For this review, take the finished solid that the model builds, in its own axes (mm). Face numbers are marked on the shaded views. A direction names the side the tool comes from. Round coordinates to 2 decimals unless told otherwise and drop trailing zeros. Write each loop counter-clockwise with the first axis right and the second up, starting at its lowest first coordinate (ties: lowest second). Pieces come first, ordered by that corner, then holes. Notation, with made-up numbers: (60, 31.25) - (100, 31.25) arc R9 ccw to (100, 38.25) - close; hole circle Ø10 at (-9, 67). An arc over 180 degrees is marked (long way). One line per item, written item: value. Start each with the question number.
Q1. Add section D-D on z = -13.5. Write out the cut boundary in (x, y), and give its area (3 significant figures).
Q2. Add section C-C on x = -16. Write out the cut boundary in (y, z), and give its area (3 significant figures).
Q3. Add section A-A on z = 0. Write out the cut boundary in (x, y), and give its area (3 significant figures).
Q4. Tool access review of the marked faces 1 and 2: name each direction out of +Z, -Z, +X, -X, +Y, -Y from which nothing blocks a thin tool from reaching the whole face with its end or side.
Q5. For probe 1 along X at (y, z) = (-2.9, 0); probe 2 along Z at (x, y) = (12, -3.35); probe 3 along X at (y, z) = (-1.5, -11), list the stretches that pass through material, from the lowest coordinate up.
Q6. Clearance check with flat-ended pins moving along their axes: pin 1 Ø3 at (x, y) = (3, -2) entering from +Z; pin 2 Ø3 at (y, z) = (-2.5, 5.5) entering from +X. State where each tip first meets the part, or that it passes through.
Q7. Add section B-B on x = 0. Write out the cut boundary in (y, z).
```python
from build123d import *
from build123d.topology import SkipClean

# Parameters (mm, degrees)
SKETCH1_W                         = 40
SKETCH1_H                         = 40
BOSS_EXTRUDE1_DEPTH               = 2
F_25_0MM_DOWEL_HOLE1_D            = 20
SKETCH9_W                         = 36
SKETCH9_H                         = 36
SKETCH9_R                         = 10
BOSS_EXTRUDE2_DEPTH               = 4
TAP_DRILL_FOR_M4_TAP2_D           = 3.3
TAP_DRILL_FOR_M4_TAP2_CSINK_D     = 4
TAP_DRILL_FOR_M4_TAP2_CSINK_ANGLE = 90


with BuildPart() as part:
    # Sketch1 → Boss-Extrude1 (new body)
    with BuildSketch(Plane(origin=(0, 0, 0), x_dir=(1, 0, 0), z_dir=(0, 1, 0))):
        Rectangle(SKETCH1_W, SKETCH1_H)
    extrude(amount=BOSS_EXTRUDE1_DEPTH)

    # 25.0mm Dowel Hole1 (through all)
    with Locations(Plane(origin=(0, 0, 0), x_dir=(-1, 0, 0), z_dir=(0, -1, 0))):
        with Locations((0, 0)):
            Hole(F_25_0MM_DOWEL_HOLE1_D / 2)

    # Sketch9 → Boss-Extrude2 (add)
    with SkipClean():  # the faces are left unmerged after this step: merging them gives an invalid solid
        with BuildSketch(Plane.XZ):
            Rectangle(SKETCH9_W, SKETCH9_H)
            with Locations(Location((0, 0, 0), (0, 0, 270))):
                Circle(SKETCH9_R, mode=Mode.SUBTRACT)
        extrude(amount=BOSS_EXTRUDE2_DEPTH)
    add(part.part.scale(1), mode=Mode.REPLACE)  # the faces are merged on a copy

    # Tap Drill for M4 Tap2 (through all)
    with Locations(Plane(origin=(0, 2, 0), x_dir=(1, 0, 0), z_dir=(0, 1, 0))):
        with Locations((-10.960155108, 10.960155108), (10.960155108, 10.960155108), (10.960155108, -10.960155108), (-10.960155108, -10.960155108)):
            CounterSinkHole(TAP_DRILL_FOR_M4_TAP2_D / 2, TAP_DRILL_FOR_M4_TAP2_CSINK_D / 2, counter_sink_angle=TAP_DRILL_FOR_M4_TAP2_CSINK_ANGLE)


solid = part.part
```
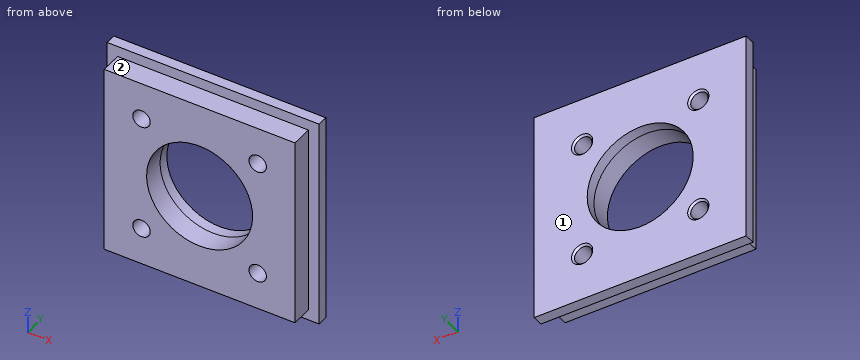
Result set:
1. outline: (-20, 0) - (-18, 0) - (-18, -4) - (18, -4) - (18, 0) - (20, 0) - (20, 2) - (-20, 2) - close
1. area: 224 mm^2
2. outline: (-4, -18) - (0, -18) - (0, -20) - (2, -20) - (2, 20) - (0, 20) - (0, 18) - (-4, 18) - close
2. area: 224 mm^2
3. outline: (-20, 0) - (-18, 0) - (-18, -4) - (-10, -4) - (-10, 2) - (-20, 2) - close; (10, -4) - (18, -4) - (18, 0) - (20, 0) - (20, 2) - (10, 2) - close
3. area: 104 mm^2
4. face 1: +Z, -Z, +X, -X, +Y
4. face 2: +Z, +X, -X, -Y
5. probe 1: x = -18 to -10, 10 to 18
5. probe 2: z = -18 to -12.24, -9.68 to 9.68, 12.24 to 18
5. probe 3: x = -18 to -12.61, -9.31 to 9.31, 12.61 to 18
6. pin 1: stops at z = 18
6. pin 2: stops at x = 18
7. outline: (-4, -18) - (0, -18) - (0, -20) - (2, -20) - (2, -10) - (-4, -10) - close; (-4, 10) - (2, 10) - (2, 20) - (0, 20) - (0, 18) - (-4, 18) - close
